```python
from build123d import *

# Parameters (mm, degrees)
BOSS_EXTRUDE1_DEPTH = 10


with BuildPart() as part:
    # Sketch1 → Boss-Extrude1 (new body)
    with BuildSketch(Plane.XY):
        with BuildLine():
            Line((-0.3, 11.729179607), (-3.2, 5.929179607))
            Line((-3.2, 5.929179607), (-3.2, -4))
            ThreePointArc((-3.2, -4), (-2.702081528, -5.202081528), (-1.5, -5.7))
            Line((-1.5, -5.7), (0, -5.7))
            Line((0, -5.7), (1.7, -5.7))
            Line((1.7, -5.7), (1.7, -0.3))
            Line((1.7, -0.3), (-0.3, -0.3))
            Line((-0.3, -0.3), (-0.3, 11.729179607))
        make_face()
    extrude(amount=BOSS_EXTRUDE1_DEPTH)


solid = part.part
```
Verification items for the finished model (mm, model axes). A direction names the side the tool comes from. Coordinates: 2 decimals unless noted, no trailing zeros. Loops run counter-clockwise (first coordinate to the right, second up) from the corner with the lowest first, then second, coordinate; pieces in that order, holes last. Notation, with made-up numbers: (63.25, 82.25) - (83.25, 82.25) arc R33 ccw to (83.25, 110.25) - close; hole circle Ø10 at (-25, 8.5). An arc over 180 degrees is marked (long way). Put each result on its own line as item: value.
Item 1: Section check C-C (y = 7.5). Enter the section's corners in (x, z).
Conclusion:
outline: (-2.41, 0) - (-0.3, 0) - (-0.3, 10) - (-2.41, 10) - close
Item 2: Section check A-A (z = 1.25). Enter the section's corners in (x, y).
Conclusion:
outline: (-3.2, -4) arc R1.7 ccw to (-1.5, -5.7) - (1.7, -5.7) - (1.7, -0.3) - (-0.3, -0.3) - (-0.3, 11.73) - (-3.2, 5.93) - close
Item 3: Set-up check for faces 1 (the face through (-0.3, 6, 5)), 2 (the face through (1.7, -3, 5)): record each of +Z, -Z, +X, -X, +Y, -Y from which the full face is reachable in a straight line by a thin tool's end or side.
Conclusion:
face 1: +Z, -Z, +X, +Y
face 2: +Z, -Z, +X, +Y, -Y
Item 4: Section check B-B (x = 0.95). Enter the section's corners in (y, z), then the cut area to 3 significant figures.
Conclusion:
outline: (-5.7, 0) - (-0.3, 0) - (-0.3, 10) - (-5.7, 10) - close
area: 54.0 mm2
Item 5: Scan lines: line 1 along X through (y, z) = (5.75, 7.5); line 2 along Y through (x, z) = (-0.1, 6.25); line 3 along Y through (x, z) = (-2.55, 1). Record each from-to range of solid material in increasing order.
Conclusion:
line 1: x = -3.2 to -0.3
line 2: y = -5.7 to -0.3
line 3: y = -5.34 to 7.23
Item 6: Gauge pin test, flat end, axial feed: pin 1 Ø4 at (y, z) = (3.5, 7.5) entering from +X. Record the tip position at first contact, or that the pin passes through.
Conclusion:
pin 1: stops at x = -0.3
